```python
from build123d import *

# Parameters (mm, degrees)
F1_DEPTH = 12.7
F2_R     = 5.08201
F3_DEPTH = 10.16
F5_DEPTH = 10.16


with BuildPart() as f1:
    # F0 (on Front) → F1 (new body)
    with BuildSketch(Plane.XZ):
        Polygon((0, 12.812912), (-9.524995, -12.596868), (9.525005, -12.596868), align=None)
    extrude(amount=F1_DEPTH)

    # F2 (on face) → F3 (join)
    with BuildSketch(Plane.XZ.offset(12.7)):
        with Locations((0, -2.427088)):
            Circle(F2_R)
    extrude(amount=F3_DEPTH)

    # F4 (on face) → F5 (cut)
    with BuildSketch(Plane.XZ.offset(22.86)):
        with BuildLine():
            ThreePointArc((0, -5.348088), (2.065459, -4.492546), (2.921, -2.427088))
            ThreePointArc((2.921, -2.427088), (2.88615, -1.97722), (2.782431, -1.538088))
            Line((2.782431, -1.538088), (-2.754014, -1.453617))
            ThreePointArc((-2.754014, -1.453617), (-2.384927, -4.113612), (0, -5.348088))
        make_face()
    extrude(amount=-F5_DEPTH, mode=Mode.SUBTRACT)


solid = f1.part
```
Verification items for the finished model (mm, model axes). A direction names the side the tool comes from. Round coordinates to 2 decimals unless told otherwise and drop trailing zeros. Write each loop counter-clockwise with the first axis right and the second up, starting at its lowest first coordinate (ties: lowest second). Pieces come first, ordered by that corner, then holes.
1. Gauge pin test, flat ends, axial feed: P1, Ø4, axis at y = -11, z = -1.5, coming from the +X side (3 decimals); P2, Ø10, axis at x = -1.5, z = 10, coming from the -Y side; P3, Ø4.5, axis at x = 1, z = -3.5, coming from the -Y side; P4, Ø5, axis at x = -5.5, z = 7.5, coming from the -Y side. Record the tip position at first contact, or that the pin passes through.
2. Section check A-A on y = -20. Enter the section's corners in (x, z), plus the area to 3 significant figures.
3. Section check B-B on z = 0.25. Enter the section's corners in (x, y).
4. Section check D-D on x = -8. Enter the section's corners in (y, z), plus the area to 3 significant figures.
5. Section check C-C on y = -1.5. Enter the section's corners in (x, z) (3 decimals), plus the area to 3 significant figures.
6. Access from +Z, -Z, +X, -X, +Y, -Y to the whole of each face (thin tool, end or side, straight path). Record for faces 4 (the flat face through (0, -12.7, -3)), 5 (the flat face through (0, -6, -12.597)).
7. Draft check along Z on faces 1 (the flat face through (0, 0, -3)), 2 (the cylindrical face through (2.887, -17.851, -1.983)), 3 (the cylindrical face through (-1.1, -17.71, -7.39)). Enter one of: +Z half, -Z half, draft (parallel to the pull), parting line (faces both ways), or undercut.
8. Scan lines: L1, parallel to Y at x = -1.5, z = 3.5; L2, parallel to Z at x = 0, y = -19.5; L3, parallel to Z at x = 1.5, y = -15.75. Record each from-to range of solid material in increasing order.
Answer:
1. P1: stops at x = 6.115
1. P2: stops at y = -12.7
1. P3: stops at y = -22.86
1. P4: passes through
2. outline: circle Ø10.16 at (0, -2.43); hole (-2.75, -1.45) arc R2.92 ccw to (0, -5.35) arc R2.92 ccw to (2.92, -2.43) arc R2.92 ccw to (2.78, -1.54) - close
2. area: 62.4 mm2
3. outline: (-4.71, -12.7) - (-4.32, -12.7) - (-4.32, -22.86) - (4.32, -22.86) - (4.32, -12.7) - (4.71, -12.7) - (4.71, 0) - (-4.71, 0) - close
4. outline: (-12.7, -12.6) - (0, -12.6) - (0, -8.53) - (-12.7, -8.53) - close
4. area: 51.7 mm2
5. outline: (-9.525, -12.597) - (9.525, -12.597) - (0, 12.813) - close
5. area: 242 mm2
6. face 4: -Y
6. face 5: -Z, +X, -X, +Y, -Y
7. face 1: draft
7. face 2: undercut
7. face 3: parting line
8. L1: y = -12.7 to 0
8. L2: z = -7.51 to -5.35, -1.5 to 2.65
8. L3: z = -7.28 to -4.93, -1.52 to 2.43
